Design review of the part shown in the three views and the two pictorial views. Dimensions are in mm from the part's minimum x, y and z. Give positions to 0.01 mm unless a question says otherwise; leave off trailing zeros. Loops run counter-clockwise (first coordinate to the right, second up) from the corner with the lowest first, then second, coordinate; pieces in that order, holes last. Notation, with made-up numbers: (-12, 28) -> (11, 28) arc R10 cw to (11, 45) -> close; hole circle Ø4 at (-38.5, 59.25). An arc over 180 degrees is marked (long way). One line per question, with ' | ' between items. Start each with the question number.
(1) Wall thickness on probe 1 along Y at (x, z) = (5, 21); probe 2 along X at (y, z) = (3.5, 8); probe 3 along Y at (x, z) = (6, 21): over which ranges is each line inside the solid? List them lowest first.
(2) Consider section B-B (x = 5). Write out the cut boundary in (y, z).
(3) Insertion check: P1, Ø8, axis at x = 14, z = 21, coming from the -Y side. The pin has a flat end and moves straight along its axis. Give the tip position at first contact, or say it passes through.
(4) Consider section D-D (x = 42). Write out the cut boundary in (y, z), and give its area (3 significant figures).
(5) Consider section A-A (y = 5). Write out the cut boundary in (x, z).
(6) Consider section C-C (z = 32). Write out the cut boundary in (x, y).
(7) Draft analysis for pull direction Z (two halves, no side actions). For the marked faces 1, 2 and 3, state which applies: +Z half, -Z half, draft (parallel to the pull), parting line (faces both ways), or undercut.
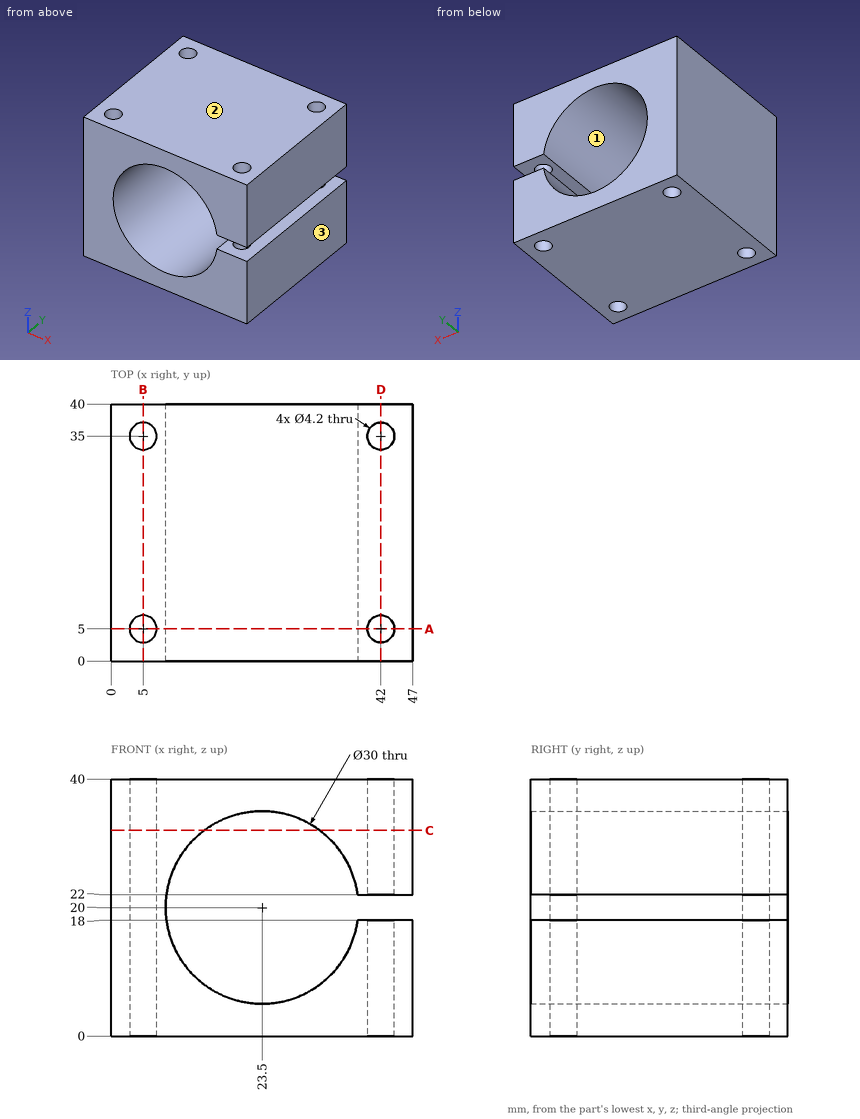
A:
1) probe 1: y = 0 to 2.9, 7.1 to 32.9, 37.1 to 40 | probe 2: x = 0 to 3.53, 6.47 to 14.5, 32.5 to 40.53, 43.47 to 47 | probe 3: y = 0 to 3.15, 6.85 to 33.15, 36.85 to 40
2) outline: (0, 0) -> (2.9, 0) -> (2.9, 40) -> (0, 40) -> close; (7.1, 0) -> (32.9, 0) -> (32.9, 40) -> (7.1, 40) -> close; (37.1, 0) -> (40, 0) -> (40, 40) -> (37.1, 40) -> close
3) P1: passes through
4) outline: (0, 0) -> (2.9, 0) -> (2.9, 18) -> (0, 18) -> close; (0, 22) -> (2.9, 22) -> (2.9, 40) -> (0, 40) -> close; (7.1, 0) -> (32.9, 0) -> (32.9, 18) -> (7.1, 18) -> close; (7.1, 22) -> (32.9, 22) -> (32.9, 40) -> (7.1, 40) -> close; (37.1, 0) -> (40, 0) -> (40, 18) -> (37.1, 18) -> close; (37.1, 22) -> (40, 22) -> (40, 40) -> (37.1, 40) -> close | area: 1,140 mm^2
5) outline: (0, 0) -> (2.9, 0) -> (2.9, 40) -> (0, 40) -> close; (7.1, 0) -> (39.9, 0) -> (39.9, 18) -> (38.37, 18) arc R15 cw (long way) to (38.37, 22) -> (39.9, 22) -> (39.9, 40) -> (7.1, 40) -> close; (44.1, 0) -> (47, 0) -> (47, 18) -> (44.1, 18) -> close; (44.1, 22) -> (47, 22) -> (47, 40) -> (44.1, 40) -> close
6) outline: (0, 0) -> (14.5, 0) -> (14.5, 40) -> (0, 40) -> close; (32.5, 0) -> (47, 0) -> (47, 40) -> (32.5, 40) -> close; hole circle Ø4.2 at (5, 5); hole circle Ø4.2 at (5, 35); hole circle Ø4.2 at (42, 5); hole circle Ø4.2 at (42, 35)
7) face 1: undercut | face 2: +Z half | face 3: draft
